The listing builds one solid part. Answer for the finished solid, in the listing's coordinates (mm). Face numbers are marked on the shaded views. A direction names the side the tool comes from. Give positions to 0.01 mm unless a question says otherwise; leave off trailing zeros. Write each loop counter-clockwise with the first axis right and the second up, starting at its lowest first coordinate (ties: lowest second). Pieces come first, ordered by that corner, then holes. Notation, with made-up numbers: (-39.75, -26.5) - (15.25, -26.5) arc R25 ccw to (15.25, 0.5) - close; hole circle Ø7 at (75.25, 54.25). An arc over 180 degrees is marked (long way). Answer in a Markdown table with one row per item. Add a question column.
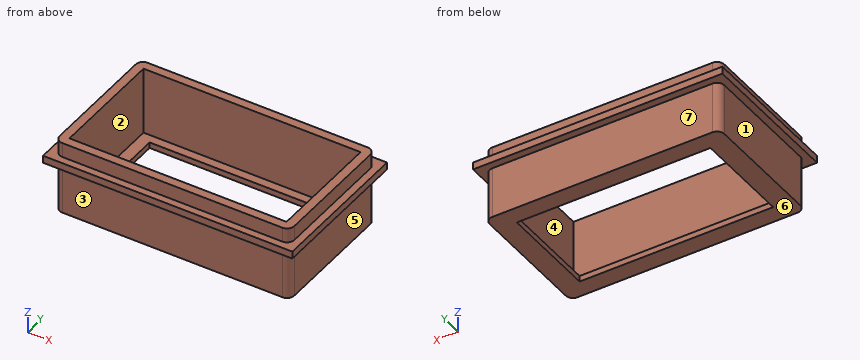
Autodesk Fusion 360 part; units mm, degrees
sketch "Sketch1" plane through (0, 0, 0) normal (0, 0, 1) x (1, 0, 0)
  line L0 (8, 4.55) -> (-8, 4.55)
  line L1 (-8, 4.55) -> (-8, -4.55)
  line L2 (-8, -4.55) -> (8, -4.55)
  line L3 (8, -4.55) -> (8, 4.55)
  line L4 (8, 4.55) -> (-8, -4.55) construction
  line L5 (-8, 4.55) -> (8, -4.55) construction
  line L6 (7.2, 3.75) -> (-7.2, 3.75)
  line L7 (-7.2, 3.75) -> (-7.2, -3.75)
  line L8 (-7.2, -3.75) -> (7.2, -3.75)
  line L9 (7.2, -3.75) -> (7.2, 3.75)
  line L10 (7.2, 3.75) -> (-7.2, -3.75) construction
  line L11 (-7.2, 3.75) -> (7.2, -3.75) construction
  line L12 (6.7, 3.35) -> (-6.7, 3.35)
  line L13 (-6.7, 3.35) -> (-6.7, -3.35)
  line L14 (-6.7, -3.35) -> (6.7, -3.35)
  line L15 (6.7, -3.35) -> (6.7, 3.35)
  line L16 (6.7, 3.35) -> (-6.7, -3.35) construction
  line L17 (-6.7, 3.35) -> (6.7, -3.35) construction
  dimension "d1" = 16
  dimension "d2" = 9.1
  dimension "d3" = 14.4
  dimension "d4" = 7.5
  dimension "d5" = 13.4
  dimension "d6" = 6.7
extrude "Extrude1" add sketch "Sketch1" along normal blind 0.2 contours L0 L1 L2 L3 | L6 L7 L8 L9
extrude "Extrude2" add sketch "Sketch1" along normal blind 5 contours L0 L1 L2 L3
fillet "Fillet1" radius 0.5 4 edges at (8, -4.55, 2.5) (-8, -4.55, 2.5) (8, 4.55, 2.5) (-8, 4.55, 2.5)
extrude "Extrude3" cut 1 faces at (7.2, 1.25, 3.4) along direction (1, 0, 0) blind 0.4
extrude "Extrude4" cut 1 faces at (-2.2667, -3.75, 1.8) along direction (0, -1, 0) blind 0.4
extrude "Extrude5" cut 1 faces at (-7.2, 1.1167, 1.8) along direction (-1, 0, 0) blind 0.4
extrude "Extrude6" cut 1 faces at (2.5333, 3.75, 1.8) along direction (0, 1, 0) blind 0.4
extrude "Extrude7" add 1 faces at (2.5333, 4.15, 1.8) along direction (0, -1, 0) blind 0.2
extrude "Extrude8" add 1 faces at (2.5333, -4.15, 3.4) along direction (0, 1, 0) blind 0.2
extrude "Extrude9" add 1 faces at (-7.6, -1.3167, 1.8) along direction (1, 0, 0) blind 0.2
extrude "Extrude10" add 1 faces at (7.6, 1.3167, 1.8) along direction (-1, 0, 0) blind 0.2
extrude "Extrude11" add 1 faces at (-7.1667, 1.1167, 0.2) along direction (0, 0, 1) blind 0.2
extrude "Extrude12" add 1 faces at (6.7, 1.1167, 0.2667) along direction (-1, 0, 0) blind 0.1
extrude "Extrude13" add 1 faces at (-6.7, 1.1167, 0.1333) along direction (1, 0, 0) blind 0.1
ref_plane "WorkPlane1" through (0, 0, 4) normal (0, 0, -1) x (-1, 0, 0)
sketch "Sketch2" plane through (0, 0, 4) normal (0, 0, -1) x (1, 0, 0)
  line L0 (8.5, -5.05) -> (-8.5, -5.05)
  line L1 (-8.5, -5.05) -> (-8.5, 5.05)
  line L2 (-8.5, 5.05) -> (8.5, 5.05)
  line L3 (8.5, 5.05) -> (8.5, -5.05)
  line L4 (8.5, -5.05) -> (-8.5, 5.05) construction
  line L5 (-8.5, -5.05) -> (8.5, 5.05) construction
  line L6 (7.5059, -4.1931) -> (-7.5059, -4.1931)
  line L7 (-7.5059, -4.1931) -> (-7.5059, 4.1931)
  line L8 (-7.5059, 4.1931) -> (7.5059, 4.1931)
  line L9 (7.5059, 4.1931) -> (7.5059, -4.1931)
  line L10 (7.5059, -4.1931) -> (-7.5059, 4.1931) construction
  line L11 (-7.5059, -4.1931) -> (7.5059, 4.1931) construction
  dimension "d36" = 17
  dimension "d37" = 10.1
extrude "Extrude14" add sketch "Sketch2" along normal blind 0.5
1. Section D-D (y = -3.75) is taken. Give the vertices of the cut face in (x, z).
2. Section A-A (y = 2.25) is taken. Give the vertices of the cut face in (x, z).
3. A tool of negligible diameter and unlimited length cuts with its end or side. For the marked faces 4, 5, 6 and 7, from which of +Z, -Z, +X, -X, +Y, -Y can it reach the whole face along a straight path? Write none if from no direction.
4. Straight lines are drawn through the part: L1, parallel to Y at x = 3.75, z = 4.55; L2, parallel to X at y = -2, z = 3.35; L3, parallel to Y at x = -6.5, z = 3.6. For each, find the intervals that lie inside material, in ascending order. Write a range as [from, to].
5. Section B-B (x = -4.5) is taken. Give the vertices of the cut face in (y, z), and give its area (3 significant figures).
6. The mould has two halves that part along Y. Classify the marked faces 1, 2 and 3: +Y half, -Y half, draft (parallel to the pull), parting line (faces both ways), or undercut.
7. Section C-C (z = 2.35) is taken. Give the vertices of the cut face in (x, y), and give its area (3 significant figures).
8. Given pin 1 Ø2 at (y, z) = (1, 0.5) entering from +X; pin 2 Ø2.5 at (x, z) = (-1, 1.5) entering from -Y; pin 3 Ø1 at (y, z) = (0, 1) entering from -X, each flat-ended and moving along its own axis, determine where each tip first touches the part or whether it passes through.
Geometry check:
| question | item | result |
|---|---|---|
| 1 | outline | (-8.5, 3.5) - (-8, 3.5) - (-8, 0) - (8, 0) - (8, 3.5) - (8.5, 3.5) - (8.5, 4) - (8, 4) - (8, 5) - (7.4, 5) - (7.4, 0.4) - (-7.4, 0.4) - (-7.4, 5) - (-8, 5) - (-8, 4) - (-8.5, 4) - close |
| 2 | outline | (-8.5, 3.5) - (-8, 3.5) - (-8, 0) - (-6.6, 0) - (-6.6, 0.4) - (-7.4, 0.4) - (-7.4, 5) - (-8, 5) - (-8, 4) - (-8.5, 4) - close; (6.6, 0) - (8, 0) - (8, 3.5) - (8.5, 3.5) - (8.5, 4) - (8, 4) - (8, 5) - (7.4, 5) - (7.4, 0.4) - (6.6, 0.4) - close |
| 3 | face 4 | +Z |
| 3 | face 5 | -Z, +X, +Y, -Y |
| 3 | face 6 | -Z, +X, -X, +Y, -Y |
| 3 | face 7 | -Z, +X, -X, +Y |
| 4 | L1 | [-4.55, -3.95], [3.95, 4.55] |
| 4 | L2 | [-8, -7.4], [7.4, 8] |
| 4 | L3 | [-5.05, -3.95], [3.95, 5.05] |
| 5 | outline | (-5.05, 3.5) - (-4.55, 3.5) - (-4.55, 0) - (-3.35, 0) - (-3.35, 0.4) - (-3.95, 0.4) - (-3.95, 5) - (-4.55, 5) - (-4.55, 4) - (-5.05, 4) - close; (3.35, 0) - (4.55, 0) - (4.55, 3.5) - (5.05, 3.5) - (5.05, 4) - (4.55, 4) - (4.55, 5) - (3.95, 5) - (3.95, 0.4) - (3.35, 0.4) - close |
| 5 | area | 6.98 mm² |
| 6 | face 1 | draft |
| 6 | face 2 | undercut |
| 6 | face 3 | -Y half |
| 7 | outline | (-8, -4.05) arc R0.5 ccw to (-7.5, -4.55) - (7.5, -4.55) arc R0.5 ccw to (8, -4.05) - (8, 4.05) arc R0.5 ccw to (7.5, 4.55) - (-7.5, 4.55) arc R0.5 ccw to (-8, 4.05) - close; hole (-7.4, -3.95) - (7.4, -3.95) - (7.4, 3.95) - (-7.4, 3.95) - close |
| 7 | area | 28.5 mm² |
| 8 | pin 1 | x = 8 |
| 8 | pin 2 | y = -4.55 |
| 8 | pin 3 | x = -8 |
